Read the model definition and answer for the solid it produces. Units are mm, in the model's axes. Face numbers are marked on the shaded views. Give positions to 0.01 mm unless a question says otherwise; leave off trailing zeros. Loops run counter-clockwise (first coordinate to the right, second up) from the corner with the lowest first, then second, coordinate; pieces in that order, holes last. Notation, with made-up numbers: (-10.75, 24) - (24.25, 24) arc R33 ccw to (24.25, 61) - close; hole circle Ø5 at (86.25, 38). An arc over 180 degrees is marked (long way). Put each result on its own line as item: value. Start each with the question number.
1. For a pull along X with two mould halves and no side action, classify the marked faces 1, 2, 3 and 4 as released by +X, released by -X, zero draft, split by the parting line, or undercut.
2. A cutting plane is placed at D-D, the plane z = 8. Determine the outline of the cut face in (x, y), plus the area to 3 significant figures.
3. Given pin 1 Ø3 at (x, y) = (-23.5, -14.5) entering from +Z; pin 2 Ø4 at (x, y) = (12.5, 26) entering from +Z; pin 3 Ø10 at (x, y) = (26, 15.5) entering from +Z, each flat-ended and moving along its own axis, determine where each tip first touches the part or whether it passes through.
4. A cutting plane is placed at B-B, the plane z = 3.5. Determine the outline of the cut face in (x, y), plus the area to 3 significant figures.
5. Consider L1, parallel to X at y = -14, z = 3; L2, parallel to X at y = -12, z = 9; L3, parallel to Z at x = -4, y = -11.5. Determine where each line is inside the solid, lowest interval first. Write a range as from..to.
```python
from build123d import *

# Parameters (mm, degrees)
F0_W        = 80
F0_H        = 80
F0_W_2      = 40
F0_H_2      = 12.5
F1_DEPTH    = 10.1
F2_T1_DEPTH = 170.5154722058
F3_SIZE2    = 19.822356
F3_SIZE     = 10.09999
F3_2_SIZE2  = 19.822356
F3_2_SIZE   = 10.09999
F4_SIZE2    = 49.643076
F4_SIZE     = 10.09999
F5_DEPTH    = 2.1


# Not quite as in the source:
# - a fillet or chamfer that OpenCascade refuses, or shapes differently, is made with other operations: its cross-section is extruded or revolved along the edge and cut away or added
# - a fillet or chamfer is up to 0.001 mm smaller than in the source, because OpenCascade refuses the exact size


with BuildPart() as f1:
    # F0 (on Top) → F1 (new body)
    with BuildSketch(Plane.XY):
        Rectangle(F0_W, F0_H)
        with Locations((0, -16.3821391761)):
            Rectangle(F0_W_2, F0_H_2, mode=Mode.SUBTRACT)
    extrude(amount=F1_DEPTH)

    # F2: chamfer of 10.1 x 17.4937131564 on 1 edges, made by hand

    # F2_s2 → F2_t1 (cut)
    with BuildSketch(Plane.YZ.offset(-85.2577361029)):
        Polygon((-40, 0), (-22.5062868436, 10.1), (-40, 10.1), align=None)
    extrude(amount=F2_T1_DEPTH, mode=Mode.SUBTRACT)

    # F3 (size 10.1 and 19.8223661056 in the source; OpenCascade refuses exactly that, so slightly less here)
    f3_edges = [f1.edges().sort_by_distance(p)[0] for p in [
        (-40, 8.746857, 10.1),
    ]]
    f3_side = f1.faces().sort_by_distance((-40, 4.194471, 4.843358))[0]
    chamfer(f3_edges, length=F3_SIZE, length2=F3_SIZE2, reference=f3_side)

    # F3#2 (size 10.1 and 19.8223661056 in the source; OpenCascade refuses exactly that, so slightly less here)
    f3_2_edges = [f1.edges().sort_by_distance(p)[0] for p in [
        (40, 8.746857, 10.1),
    ]]
    f3_2_side = f1.faces().sort_by_distance((40, 4.194471, 4.843358))[0]
    chamfer(f3_2_edges, length=F3_2_SIZE, length2=F3_2_SIZE2, reference=f3_2_side)

    # F4 (size 10.1 and 49.6430860138 in the source; OpenCascade refuses exactly that, so slightly less here)
    f4_edges = [f1.edges().sort_by_distance(p)[0] for p in [
        (0, 40, 10.1),
    ]]
    f4_side = f1.faces().sort_by_distance((0, 40, 4.495514))[0]
    chamfer(f4_edges, length=F4_SIZE, length2=F4_SIZE2, reference=f4_side)

    # F0 (on Top) → F5 (join)
    with BuildSketch(Plane.XY):
        with Locations((0, -16.3821391761)):
            Rectangle(F0_W_2, F0_H_2)
    extrude(amount=F5_DEPTH)


solid = f1.part
```
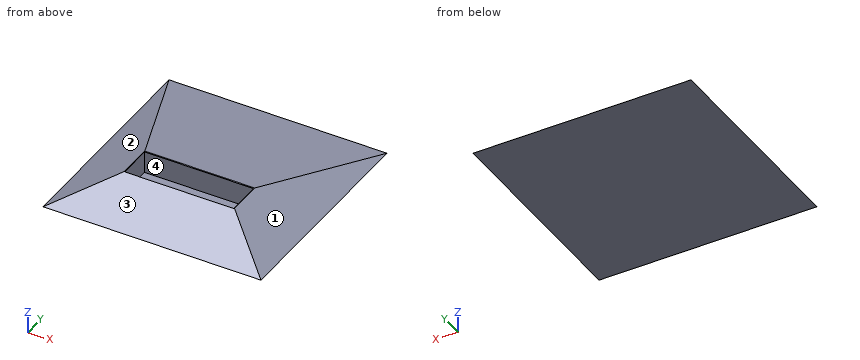
Return value:
1. face 1: released by +X
1. face 2: released by -X
1. face 3: zero draft
1. face 4: undercut
2. outline: (-24.3, -26.14) - (24.3, -26.14) - (24.3, 0.68) - (-24.3, 0.68) - close; hole (-20, -22.63) - (20, -22.63) - (20, -10.13) - (-20, -10.13) - close
2. area: 804 mm2
3. pin 1: stops at z = 9.17
3. pin 2: stops at z = 3.26
3. pin 3: stops at z = 6
4. outline: (-33.13, -33.94) - (33.13, -33.94) - (33.13, 22.8) - (-33.13, 22.8) - close; hole (-20, -22.63) - (20, -22.63) - (20, -10.13) - (-20, -10.13) - close
4. area: 3,260 mm2
5. L1: x = -34.11..-20, 20..34.11
5. L2: x = -22.34..-20, 20..22.34
5. L3: z = 0..2.1
